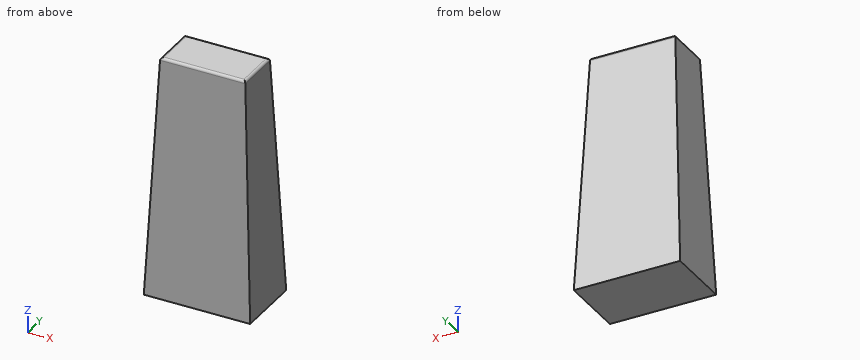
Autodesk Inventor part; units mm, degrees
ref_plane "YZ Plane" through (0, 0, 0) normal (1, 0, 0) x (0, 1, 0)
ref_plane "XZ Plane" through (0, 0, 0) normal (0, 1, 0) x (-1, 0, 0)
ref_plane "XY Plane" through (0, 0, 0) normal (0, 0, 1) x (1, 0, 0)
sketch "Sketch1" plane through (0, 0, 0) normal (0, 0, 1) x (1, 0, 0)
  line L0 (-20, 12.5) -> (20, 12.5)
  line L1 (20, 12.5) -> (20, -12.5)
  line L2 (20, -12.5) -> (-20, -12.5)
  line L3 (-20, -12.5) -> (-20, 12.5)
  point P0 (0, 0)
  dimension "d0" = 40
  dimension "d1" = 25
  dimension "d2" = 12.5
  dimension "d3" = 20
extrude "Extrusion1" add sketch "Sketch1" along normal blind 90
chamfer "Chamfer1" distance 4 distance2 90 1 edges at (0, 12.5, 90) measured on face at (-6.6667, 4.1667, 90)
chamfer "Chamfer2" distance 4 distance2 90 1 edges at (0, -12.5, 90) measured on face at (-6.6667, 1.5003, 90)
chamfer "Chamfer3" distance 4 distance2 90 1 edges at (20, 0, 90) measured on face at (-6.6667, 2.8335, 90)
chamfer "Chamfer4" distance 4 distance2 90 1 edges at (-20, 0, 90) measured on face at (-7.9998, 2.8335, 90)
fillet "Fillet1" radius 1 4 edges at (0, 8.5005, 90) (-16.0005, 0, 90) (0, -8.5005, 90) (16.0005, 0, 90)
properties part number "Foot"
Here's how the part is built. I have some questions about the finished solid (model axes, mm). Give positions to 0.01 mm unless a question says otherwise; leave off trailing zeros. Order: outer loops, then holes, each group sorted by start corner. A loop starts at its lowest first (then second) coordinate and runs counter-clockwise, first axis right, second up. Notation, with made-up numbers: M 66.25,85.5 L 101.25,85.5 A9 cw 101.25,92.5 Z; hole C -30,-25.75 d10. An arc over 180 degrees is marked long. Use a Markdown table: item, result. Add a question column.
1. For pin 1 Ø1 at (y, z) = (7, 26.5) entering from +X; pin 2 Ø10 at (x, y) = (15, -10) entering from -Z; pin 3 Ø3 at (y, z) = (7, 67.5) entering from -X; pin 4 Ø10 at (x, z) = (-11.5, 9) entering from +Y, each with a flat end and sliding along its axis, tell me the tip position at first contact or that it passes through.
2. Suppose I cut it at C-C (z = 41). List the corners of the cut face in (x, y) for me, and give its area (3 significant figures).
3. I need wall thicknesses on probe 1 along Y at (x, z) = (2.5, 80.5); probe 2 along Y at (x, z) = (-15.5, 36.5); probe 3 along X at (y, z) = (7, 54). Which ranges of each line are inside material? Lowest first, please. Write a range as from..to.
Results list:
| question | item | result |
|---|---|---|
| 1 | pin 1 | stops at x = 18.84 |
| 1 | pin 2 | stops at z = 0 |
| 1 | pin 3 | stops at x = -17.07 |
| 1 | pin 4 | stops at y = 12.32 |
| 2 | outline | M -18.18,-10.68 L 18.18,-10.68 L 18.18,10.68 L -18.18,10.68 Z |
| 2 | area | 776 mm² |
| 3 | probe 1 | y = -8.92..8.92 |
| 3 | probe 2 | y = -10.88..10.88 |
| 3 | probe 3 | x = -17.6..17.6 |
